Geometry check sheet. Reference: the model listing, model coordinates, mm. Face numbers are marked on the shaded views. A direction names the side the tool comes from. Coordinates: 2 decimals unless noted, no trailing zeros. Order: outer loops, then holes, each group sorted by start corner. A loop starts at its lowest first (then second) coordinate and runs counter-clockwise, first axis right, second up. Notation, with made-up numbers: (-21, 61) - (-17, 61) arc R34 ccw to (-17, 94) - close; hole circle Ø7 at (-25.75, 23.25). An arc over 180 degrees is marked (long way). Return JSON: item names as keys, results as strings. Group by question number.
Item 1: Tool access check on the marked faces 1, 2 and 3. Record the directions out of +Z, -Z, +X, -X, +Y, -Y that give a thin tool (end or side, any length) a straight path to the whole face; none if there is none.
Item 2: Section check D-D on y = 45.5. Enter the section's corners in (x, z).
Item 3: Section check B-B on x = -12.5. Enter the section's corners in (y, z), then the cut area to 3 significant figures.
Item 4: Section check A-A on z = 27.5. Enter the section's corners in (x, y), then the cut area to 3 significant figures.
Item 5: Gauge pin test, flat ends, axial feed: pin 1 (21.5 mm diameter, centred on x = 15, y = -62, fed in from +Z); pin 2 (8 mm diameter, centred on x = 11.5, y = 29, fed in from +Z); pin 3 (4 mm diameter, centred on y = 20.5, z = -6.5, fed in from -X). Record the tip position at first contact, or that the pin passes through.
Item 6: Section check C-C on y = -67. Enter the section's corners in (x, z).
Item 7: Scan lines: probe 1 along X at (y, z) = (-50.5, 26); probe 2 along Z at (x, y) = (-1, 46); probe 3 along X at (y, z) = (-40.5, 20.5). Record each from-to range of solid material in increasing order.
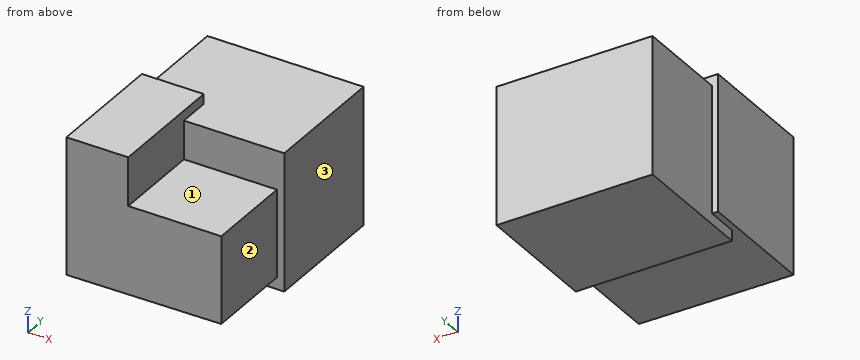
from build123d import *

# Parameters (mm, degrees)
F0_W     = 62.537648
F0_H     = 53.085398
F0_W_2   = 62.155746
F1_DEPTH = 25.4
F2_DEPTH = 76.2
F4_DEPTH = 96.774


with BuildPart() as f1:
    # F0 (on Front) → F1 (new body)
    with BuildSketch(Plane.XZ):
        Polygon((62.155746, 0), (0, 0), (-62.537648, 0), (-62.537648, -56.904487), (62.155746, -56.904487), align=None)
        with Locations((-31.268824, 26.542699)):
            Rectangle(F0_W, F0_H)
        with Locations((31.077873, 26.542699)):
            Rectangle(F0_W_2, F0_H)
    extrude(amount=F1_DEPTH)

    # F0 (on Front) → F2 (join)
    with BuildSketch(Plane.XZ):
        Polygon((62.155746, 0), (0, 0), (-62.537648, 0), (-62.537648, -56.904487), (62.155746, -56.904487), align=None)
        with Locations((-31.268824, 26.542699)):
            Rectangle(F0_W, F0_H)
        with Locations((31.077873, 26.542699)):
            Rectangle(F0_W_2, F0_H)
    extrude(amount=-F2_DEPTH)

    # F3 (on Front) → F4 (join)
    with BuildSketch(Plane.XZ):
        Polygon((-67.348078, 60.978152), (-67.348078, -48.378654), (56.28676, -47.44057), (56.28676, 22.282878), (-18.005297, 22.282878), (-18.005297, 60.978152), align=None)
    extrude(amount=F4_DEPTH)


solid = f1.part
Computed:
{
 "1": {"face 1": "+Z, +X, -Y", "face 2": "+Z, -Z, +X, -Y", "face 3": "+Z, -Z, +X, +Y, -Y"},
 "2": {"outline": "(-62.54, -56.9) - (62.16, -56.9) - (62.16, 53.09) - (-62.54, 53.09) - close"},
 "3": {"outline": "(-96.77, -47.96) - (-25.4, -47.96) - (-25.4, -56.9) - (76.2, -56.9) - (76.2, 53.09) - (-25.4, 53.09) - (-25.4, 22.28) - (-96.77, 22.28) - close", "area": "16,200 mm²"},
 "4": {"outline": "(-67.35, -96.77) - (-18.01, -96.77) - (-18.01, -25.4) - (62.16, -25.4) - (62.16, 76.2) - (-62.54, 76.2) - (-62.54, 0) - (-67.35, 0) - close", "area": "16,300 mm²"},
 "5": {"pin 1": "stops at z = 22.28", "pin 2": "stops at z = 53.09", "pin 3": "stops at x = -62.54"},
 "6": {"outline": "(-67.35, -48.38) - (56.29, -47.44) - (56.29, 22.28) - (-18.01, 22.28) - (-18.01, 60.98) - (-67.35, 60.98) - close"},
 "7": {"probe 1": "x = -67.35 to -18.01", "probe 2": "z = -56.9 to 53.09", "probe 3": "x = -67.35 to 56.29"}
}
